The listing builds one solid part. Answer for the finished solid, in the listing's coordinates (mm). A direction names the side the tool comes from. Round coordinates to 2 decimals unless told otherwise and drop trailing zeros. Write each loop counter-clockwise with the first axis right and the second up, starting at its lowest first coordinate (ties: lowest second). Pieces come first, ordered by that corner, then holes. Notation, with made-up numbers: M -25,29 L 15,29 A21 ccw 15,48 Z; hole C 46.25,-29.5 d10. An arc over 180 degrees is marked long. One line per item, written item: value. Start each with the question number.
(1) For faces 1 (the flat face through (-2, -9, 75)), 2 (the flat face through (-2, 0, 78)), determine the directions among +Z, -Z, +X, -X, +Y, -Y from which every point of the face is accessible in a straight line to the end or side of a thin tool.
(2) For a pull along Z with two mould halves and no side action, classify faces 3 (the flat face through (145, -9, -2)), 4 (the flat face through (-2, -9, -75)), 5 (the flat face through (-2, -9, 115)), 6 (the flat face through (-2, -9, -115)) as released by +Z, released by -Z, zero draft, split by the parting line, or undercut.
(3) Consider probe 1 along Z at (x, y) = (71.5, -3.5); probe 2 along X at (y, z) = (-4, -43.5). Determine where each line is inside the solid, lowest interval first.
(4) Section B-B (x = 78.5) is taken. Determine the outline of the cut face in (y, z).
(5) Section A-A (z = 18) is taken. Determine the outline of the cut face in (x, y).
(6) Section C-C (y = -9.25) is taken. Determine the outline of the cut face in (x, z).
```python
from build123d import *

# Parameters (mm, degrees)
F0_W     = 290
F0_H     = 230
F2_DEPTH = 19
F1_W     = 215
F1_H     = 150
F3_DEPTH = 25


with BuildPart() as f2:
    # F0 (on Front) → F2 (new body)
    with BuildSketch(Plane.XZ):
        Rectangle(F0_W, F0_H)
    extrude(amount=F2_DEPTH)

    # F1 (on face) → F3 (cut)
    with BuildSketch(Plane.XZ):
        Rectangle(F1_W, F1_H)
    extrude(amount=F3_DEPTH, mode=Mode.SUBTRACT)


solid = f2.part
```
Recorded:
1. face 1: +Y, -Y
1. face 2: +Z, -Z, +X, -X, +Y
2. face 3: zero draft
2. face 4: undercut
2. face 5: released by +Z
2. face 6: released by -Z
3. probe 1: z = -115 to -75, 75 to 115
3. probe 2: x = -145 to -107.5, 107.5 to 145
4. outline: M -19,-115 L 0,-115 L 0,-75 L -19,-75 Z; M -19,75 L 0,75 L 0,115 L -19,115 Z
5. outline: M -145,-19 L -107.5,-19 L -107.5,0 L -145,0 Z; M 107.5,-19 L 145,-19 L 145,0 L 107.5,0 Z
6. outline: M -145,-115 L 145,-115 L 145,115 L -145,115 Z; hole M -107.5,-75 L 107.5,-75 L 107.5,75 L -107.5,75 Z
